Can you work these out from the model? Positions are in its coordinate system, mm. A direction names the side the tool comes from. Coordinates: 2 decimals unless noted, no trailing zeros. Order: outer loops, then holes, each group sorted by start corner. A loop starts at its lowest first (then second) coordinate and runs counter-clockwise, first axis right, second up. Notation, with made-up numbers: (0.5, 34) -> (20.5, 34) arc R13 cw to (20.5, 50) -> close; hole circle Ø7 at (43, 45). An arc over 180 degrees is marked (long way). Answer as CSV lines item,"result".
from build123d import *

# Parameters (mm, degrees)
SKETCH_1_W                      = 120
SKETCH_1_H                      = 20
EXTRUDE_1_DEPTH                 = 25
CUT_EXTRUDE_1_DEPTH             = 30
SKETCH_3_W                      = 15
SKETCH_3_H                      = 25
SKETCH_3_W_2                    = 70.609699787
CUT_EXTRUDE_2_DEPTH             = 30
HOLE_WIZARD_G1_16_1_D           = 6.6
HOLE_WIZARD_G1_16_1_DEPTH       = 30
HOLE_WIZARD_G1_16_1_CSINK_D     = 7.773
HOLE_WIZARD_G1_16_1_CSINK_ANGLE = 90
HOLE_WIZARD_G1_16_1_TIP         = 1.982840043
HOLE_WIZARD_G1_16_2_D           = 6.6
HOLE_WIZARD_G1_16_2_DEPTH       = 30
HOLE_WIZARD_G1_16_2_CSINK_D     = 7.773
HOLE_WIZARD_G1_16_2_CSINK_ANGLE = 90
HOLE_WIZARD_G1_16_2_TIP         = 1.982840043


with BuildPart() as part:
    # 草图1 → 凸台-拉伸1 (new body)
    with BuildSketch(Plane(origin=(0, 0, 0), x_dir=(1, 0, 0), z_dir=(0, 1, 0))):
        with Locations((10.609699787, 0.249516379)):
            Rectangle(SKETCH_1_W, SKETCH_1_H)
    extrude(amount=EXTRUDE_1_DEPTH)

    # 草图2 → 切除-拉伸1 (cut)
    with BuildSketch(Plane.ZY.offset(49.390300213)):
        Polygon((-10.249516379, 12.5), (-10.249516379, 21.5), (9.750483621, 21.5), (9.750483621, 3.5), (-10.249516379, 3.5), align=None)
    extrude(amount=-CUT_EXTRUDE_1_DEPTH, mode=Mode.SUBTRACT)

    # 草图3 → 切除-拉伸2 (cut)
    with BuildSketch(Plane.XY.offset(9.750483621)):
        with Locations((-7.5, 12.5)):
            Rectangle(SKETCH_3_W, SKETCH_3_H)
        with Locations((35.304849894, 12.5)):
            Rectangle(SKETCH_3_W_2, SKETCH_3_H)
    extrude(amount=-CUT_EXTRUDE_2_DEPTH, mode=Mode.SUBTRACT)

    # G1/16 螺纹孔1
    with Locations(Plane(origin=(0, 25, 0), x_dir=(1, 0, 0), z_dir=(0, 1, 0))):
        with Locations((-36.390300213, 0.249516379)):
            CounterSinkHole(HOLE_WIZARD_G1_16_1_D / 2, HOLE_WIZARD_G1_16_1_CSINK_D / 2, depth=HOLE_WIZARD_G1_16_1_DEPTH, counter_sink_angle=HOLE_WIZARD_G1_16_1_CSINK_ANGLE)
            with Locations((0, 0, -(HOLE_WIZARD_G1_16_1_DEPTH + HOLE_WIZARD_G1_16_1_TIP / 2))):  # 118° drill point
                Cone(0, HOLE_WIZARD_G1_16_1_D / 2, HOLE_WIZARD_G1_16_1_TIP, mode=Mode.SUBTRACT)

    # G1/16 螺纹孔2
    with Locations(Plane.ZY.offset(19.390300213)):
        with Locations((0, 12.5)):
            CounterSinkHole(HOLE_WIZARD_G1_16_2_D / 2, HOLE_WIZARD_G1_16_2_CSINK_D / 2, depth=HOLE_WIZARD_G1_16_2_DEPTH, counter_sink_angle=HOLE_WIZARD_G1_16_2_CSINK_ANGLE)
            with Locations((0, 0, -(HOLE_WIZARD_G1_16_2_DEPTH + HOLE_WIZARD_G1_16_2_TIP / 2))):  # 118° drill point
                Cone(0, HOLE_WIZARD_G1_16_2_D / 2, HOLE_WIZARD_G1_16_2_TIP, mode=Mode.SUBTRACT)


solid = part.part
Q1. If I drill on line 1 (Y direction, x = -25, z = 6.75); line 2 (Y direction, x = -15.9, z = 0); line 3 (Z direction, x = -16.05, y = 12.5), over which ranges is the centre line in solid material (lowest first)?
Solution:
line 1,"0 to 3.5, 21.5 to 25"
line 2,"0 to 9.2, 15.8 to 25"
line 3,"-10.25 to -3.3, 3.3 to 9.75"
Q2. Imagine slicing it at D-D (z = -1.75). Give the number of separate pieces and of enclosed holes in the cut face, and give its area (3 significant figures).
Solution:
separate pieces,"4"
enclosed holes,"0"
area,"253 mm2"
Q3. Imagine slicing it at C-C (z = 8). List the corners of the cut face in (x, y) for me.
Solution:
outline,"(-49.39, 0) -> (-15, 0) -> (-15, 25) -> (-49.39, 25) -> (-49.39, 21.5) -> (-19.39, 21.5) -> (-19.39, 3.5) -> (-49.39, 3.5) -> close"
Q4. Which directions (+Z, -Z, +X, -X, +Y, -Y) give clear straight access to the entire face, cutting with the end or side of a thin tool? Please do faces 1 (the flat face through (-49.39, 23, 0)), 2 (the flat face through (-31, 3.5, 0)).
Solution:
face 1,"+Z, -Z, -X, +Y, -Y"
face 2,"+Z, -Z, -X"
Q5. Imagine slicing it at B-B (x = -44). List the corners of the cut face in (y, z) for me, and give its area (3 significant figures).
Solution:
outline,"(0, -10.25) -> (3.5, -10.25) -> (3.5, 9.75) -> (0, 9.75) -> close; (21.5, -10.25) -> (25, -10.25) -> (25, 9.75) -> (21.5, 9.75) -> close"
area,"140 mm2"
Q6. For P1, Ø5.5, axis at y = 10.5, z = -0.5, coming from the -X side; P2, Ø7.5, axis at x = -36.39, z = -0.25, coming from the +Y side; P3, Ø6, axis at x = -38.5, z = -3, coming from the +Y side; P4, Ø7.5, axis at y = 12.5, z = 0, coming from the -X side, each with a flat end and sliding along its axis, tell me the tip position at first contact or that it passes through.
Solution:
P1,"x = -19.39"
P2,"y = 24.86"
P3,"y = 25"
P4,"x = -19.25"
Q7. We'd pull the mould along X, two halves only. Please class faces 3 (the cylindrical face through (-33.772, 1.726, 1.758)), 4 (the cylindrical face through (-33.772, 22.936, 1.758)), 5 (the flat face through (-31, 21.5, 0)), 6 (the flat face through (-49.39, 2, 0)): pulls with the +X half, pulls with the -X half, needs draft (parallel to the pull), parting line crosses it, or undercut.
Solution:
face 3,"undercut"
face 4,"undercut"
face 5,"needs draft"
face 6,"pulls with the -X half"
Q8. Imagine slicing it at A-A (y = 12.5). List the corners of the cut face in (x, z) for me.
Solution:
outline,"(-19.39, -10.25) -> (-15, -10.25) -> (-15, -3.3) -> (-18.8, -3.3) -> (-19.39, -3.89) -> close; (-19.39, 3.89) -> (-18.8, 3.3) -> (-15, 3.3) -> (-15, 9.75) -> (-19.39, 9.75) -> close"
